Autodesk Inventor part; units mm, degrees
ref_plane "YZ Plane" through (0, 0, 0) normal (1, 0, 0) x (0, 1, 0)
ref_plane "XZ Plane" through (0, 0, 0) normal (0, 1, 0) x (-1, 0, 0)
ref_plane "XY Plane" through (0, 0, 0) normal (0, 0, 1) x (1, 0, 0)
sketch "스케치1" plane through (0, 0, 0) normal (0, 1, 0) x (-1, 0, 0)
  line L0 (17.6385, -30.5508) -> (-17.6385, -30.5508)
  line L1 (-17.6385, -30.5508) -> (-35.277, 0)
  line L2 (-35.277, 0) -> (-17.6385, 30.5508)
  line L3 (-17.6385, 30.5508) -> (17.6385, 30.5508)
  line L4 (17.6385, 30.5508) -> (35.277, 0)
  line L5 (35.277, 0) -> (17.6385, -30.5508)
  line L6 (19.486, -33.7508) -> (-19.486, -33.7508)
  line L7 (-19.486, -33.7508) -> (-38.972, 0)
  line L8 (-38.972, 0) -> (-19.486, 33.7508)
  line L9 (-19.486, 33.7508) -> (19.486, 33.7508)
  line L10 (19.486, 33.7508) -> (38.972, 0)
  line L11 (38.972, 0) -> (19.486, -33.7508)
  point P0 (0, 0)
  point P1 (0, 0)
  point P2 (0, 0)
  dimension "d0" = 70.554
  dimension "d1" = 3.2
extrude "돌출1" add sketch "스케치1" along normal blind 4.4 contours L0 L1 L2 L3 L4 L5 | L6 L7 L8 L9 L10 L11
sketch "스케치2" plane through (0, 4.4, 0) normal (0, 1, 0) x (1, 0, 0)
  line L0 (-18.5623, 32.1508) -> (18.5623, 32.1508)
  line L1 (18.5623, 32.1508) -> (37.1245, 0)
  line L2 (37.1245, 0) -> (18.5623, -32.1508)
  line L3 (18.5623, -32.1508) -> (-18.5623, -32.1508)
  line L4 (-18.5623, -32.1508) -> (-37.1245, 0)
  line L5 (-37.1245, 0) -> (-18.5623, 32.1508)
  line L6 (-19.486, 33.7508) -> (-38.972, 0)
  point P0 (0, 0)
  point P1 (0, 0)
  dimension "d4" = 1.6
extrude "돌출2" cut sketch "스케치2" against normal blind 1.2
sketch "스케치3" plane through (0, 3.2, 0) normal (0, 1, 0) x (1, 0, 0)
  line L0 (17.4076, -30.1508) -> (-17.4076, -30.1508)
  line L1 (-17.4076, -30.1508) -> (-34.8151, 0)
  line L2 (-34.8151, 0) -> (-17.4076, 30.1508)
  line L3 (-17.4076, 30.1508) -> (17.4076, 30.1508)
  line L4 (17.4076, 30.1508) -> (34.8151, 0)
  line L5 (34.8151, 0) -> (17.4076, -30.1508)
  line L6 (-18.5623, 32.1508) -> (18.5623, 32.1508)
  point P0 (0, 0)
  point P1 (0, 0)
  dimension "d7" = 2
extrude "돌출3" add sketch "스케치3" along normal blind 0.6
fillet "모깎기1" radius 1.2 12 edges at (0, 4.4, -33.7508) (0, 0, -33.7508) (-29.229, 4.4, -16.8754) (-29.229, 0, -16.8754) (-29.229, 4.4, 16.8754) (-29.229, 0, 16.8754) (0, 0, 33.7508) (0, 4.4, 33.7508) (29.229, 0, 16.8754) (29.229, 4.4, 16.8754) (29.229, 4.4, -16.8754) (29.229, 0, -16.8754)
sketch "스케치4" plane through (0, 0, 0) normal (0, -1, 0) x (1, 0, 0)
  line L0 (10, -7.5) -> (-10, -7.5)
  line L1 (-10, -7.5) -> (-10, -2.5)
  line L2 (-10, -2.5) -> (10, -2.5)
  line L3 (10, -2.5) -> (10, -7.5)
  line L4 (10, -7.5) -> (-10, -2.5) construction
  line L5 (-10, -7.5) -> (10, -2.5) construction
  line L6 (10, 2.5) -> (-10, 2.5)
  line L7 (-10, 2.5) -> (-10, 7.5)
  line L8 (-10, 7.5) -> (10, 7.5)
  line L9 (10, 7.5) -> (10, 2.5)
  line L10 (10, 2.5) -> (-10, 7.5) construction
  line L11 (-10, 2.5) -> (10, 7.5) construction
  point P0 (0, 0)
  point P1 (0, -5)
  point P2 (0, 5)
  dimension "d11" = 20
  dimension "d12" = 5
  dimension "d13" = 20
  dimension "d14" = 5
  dimension "d16" = 5
  dimension "d17" = 2.5
extrude "돌출4" add sketch "스케치4" along normal blind 10
sketch "스케치5" plane through (10, 0, -7.5) normal (0, 0, -1) x (-1, 0, 0)
  circle A0 centre (15, -5) radius 1.25
  circle A1 centre (5, -5) radius 1.25
  line L0 (0, 0) -> (0, -10)
  line L1 (-8.7932, 0) -> (28.7932, 0)
  point P0 (10, 0)
  point P1 (0, -5)
  dimension "d20" = 2.5
  dimension "d21" = 2.5
  dimension "d22" = 5
  dimension "d23" = 5
  dimension "d24" = 10
extrude "돌출5" cut sketch "스케치5" against normal up to surface (15 mm away)
properties part number "OV-PAM_n_6_bottom"
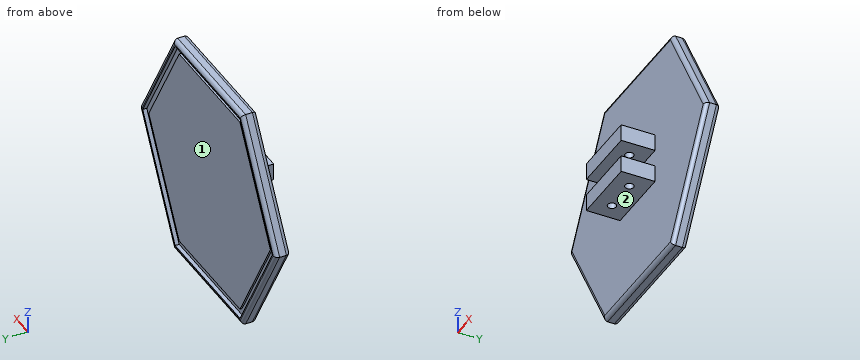
Verification items for the finished model (mm, model axes). Face numbers are marked on the shaded views. Give positions to 0.01 mm unless a question says otherwise; leave off trailing zeros. Order: outer loops, then holes, each group sorted by start corner. A loop starts at its lowest first (then second) coordinate and runs counter-clockwise, first axis right, second up. Notation, with made-up numbers: M 26.5,5 L 54.5,5 A17 cw 54.5,14 Z; hole C 9,-7 d10. An arc over 180 degrees is marked long. Return JSON: item names as keys, results as strings. Group by question number.
1) Section check A-A on y = -5. Record the cut outline in (x, z).
2) Mould release check, pull along X, two halves, no side actions. Record for the marked faces 1 and 2: pulls with the +X half, pulls with the -X half, needs draft (parallel to the pull), parting line crosses it, or undercut.
3) Go/stop test with flat-tipped pins: pin 1 Ø3 at (x, y) = (-5, -5) entering from -Z; pin 2 Ø2.5 at (y, z) = (-7, 5.5) entering from +X; pin 3 Ø1.5 at (y, z) = (-7.5, -4.5) entering from -X. Record where each tip stops, or that it passes through.
4) Section check B-B on x = 5. Give the number of separate pieces and of enclosed holes in the cut face, and give its area (3 significant figures).
5) Scan lines: line 1 (Y direction, x = 5, z = -4.05); line 2 (Z direction, x = -4.5, y = -9); line 3 (Y direction, x = 20, z = 2). Record each from-to range of solid material in increasing order.
Answer block:
{
 "1": {"outline": "M -10,-7.5 L -6.25,-7.5 L -6.25,-2.5 L -10,-2.5 Z; M -10,2.5 L -6.25,2.5 L -6.25,7.5 L -10,7.5 Z; M -3.75,-7.5 L 3.75,-7.5 L 3.75,-2.5 L -3.75,-2.5 Z; M -3.75,2.5 L 3.75,2.5 L 3.75,7.5 L -3.75,7.5 Z; M 6.25,-7.5 L 10,-7.5 L 10,-2.5 L 6.25,-2.5 Z; M 6.25,2.5 L 10,2.5 L 10,7.5 L 6.25,7.5 Z"},
 "2": {"face 1": "undercut", "face 2": "needs draft"},
 "3": {"pin 1": "stops at z = -7.5", "pin 2": "stops at x = 10", "pin 3": "stops at x = -10"},
 "4": {"separate pieces": "3", "enclosed holes": "0", "area": "330 mm^2"},
 "5": {"line 1": "y = -10 to -6.25, -3.75 to 3.8", "line 2": "z = -7.5 to -2.5, 2.5 to 7.5", "line 3": "y = 0 to 3.8"}
}
